Geometry: see drawing. Coordinates: mm, zero at the bounding-box minimum. Give positions to 0.01 mm unless a question says otherwise; leave off trailing zeros. Write each loop counter-clockwise with the first axis right and the second up, starting at its lowest first coordinate (ties: lowest second). Pieces come first, ordered by that corner, then holes. Notation, with made-up numbers: (48, 8) - (81, 8) arc R35 ccw to (81, 43) - close; hole circle Ø4 at (76, 9). An arc over 180 degrees is marked (long way). Return JSON: item names as keys, results as strings.
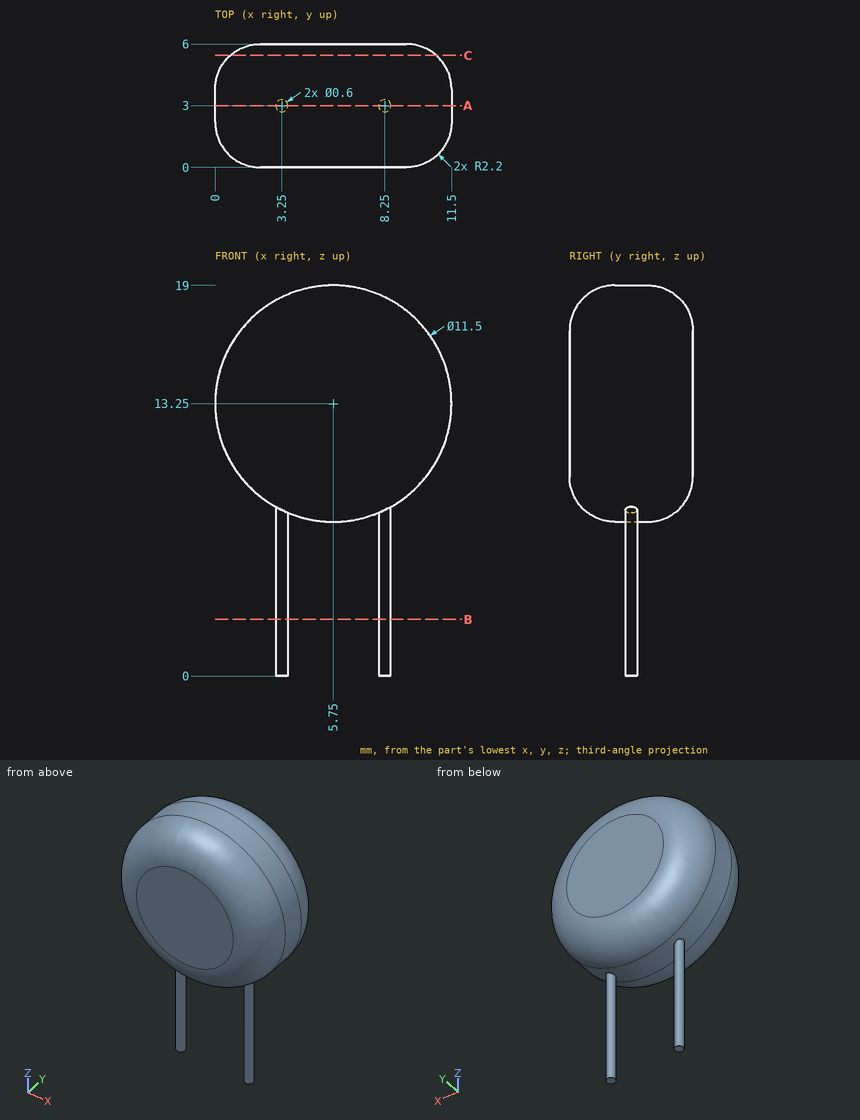
Q1. Section query C-C, the plane y = 5.45. Return the cut outline in (x, z), plus the area to 3 significant figures.
Answer key:
{"outline": "circle Ø10.01 at (5.75, 13.25)", "area": "78.7 mm^2"}
Q2. Section query B-B, the plane z = 2.75. Return the cut outline in (x, y).
Answer key:
{"outline": "circle Ø0.6 at (3.25, 3); circle Ø0.6 at (8.25, 3)"}
Q3. Section query A-A, the plane y = 3. Return the cut outline in (x, z), plus the area to 3 significant figures.
Answer key:
{"outline": "(2.95, 0) - (3.55, 0) - (3.55, 7.94) arc R5.75 ccw to (7.95, 7.94) - (7.95, 0) - (8.55, 0) - (8.55, 8.23) arc R5.75 ccw (long way) to (2.95, 8.23) - close", "area": "114 mm^2"}
Q4. Material intervals for probe 1 along Z at (x, y) = (10.5, 5.15); probe 2 along Y at (x, z) = (4.25, 17.5); probe 3 along X at (y, z) = (1.6, 11), sorted ascending. Write a range as [from, to].
Answer key:
{"probe 1": "z = [10.93, 15.57]", "probe 2": "y = [0.22, 5.78]", "probe 3": "x = [0.55, 10.95]"}
Q5. Pin query (flat end, axial travel): P1, Ø1.5, axis at x = 3.5, z = 8, coming from the +Y side; P2, Ø3, axis at y = 5.5, z = 12, coming from the +X side; P3, Ø1.5, axis at x = 3, z = 5.5, coming from the +Y side. Return the tip coordinate at first contact, or that it passes through.
Answer key:
{"P1": "stops at y = 5.49", "P2": "stops at x = 11.44", "P3": "stops at y = 3.3"}
